from build123d import *

# Parameters (mm, degrees)
SKETCH_R   = 4.3
SKETCH_R_2 = 3.3
PAD_DEPTH  = 8


with BuildPart() as part:
    # Sketch → Pad (new body)
    with BuildSketch(Plane.XY):
        with BuildLine():
            Line((180, 10), (180, 490))
            ThreePointArc((180, 490), (177.071068, 497.071068), (170, 500))
            Line((10, 500), (170, 500))
            ThreePointArc((10, 500), (2.928932, 497.071068), (0, 490))
            Line((0, 490), (0, 10))
            ThreePointArc((0, 10), (2.928932, 2.928932), (10, 0))
            Line((10, 0), (170, 0))
            ThreePointArc((170, 0), (177.071068, 2.928932), (180, 10))
        make_face()
        with Locations((75, 318)):
            Circle(SKETCH_R, mode=Mode.SUBTRACT)
        with Locations((105, 318)):
            Circle(SKETCH_R, mode=Mode.SUBTRACT)
        with Locations((105, 299)):
            Circle(SKETCH_R, mode=Mode.SUBTRACT)
        with Locations((75, 299)):
            Circle(SKETCH_R, mode=Mode.SUBTRACT)
        with Locations((20, 20)):
            Circle(SKETCH_R_2, mode=Mode.SUBTRACT)
        with Locations((20, 75)):
            Circle(SKETCH_R_2, mode=Mode.SUBTRACT)
        with Locations((20, 130)):
            Circle(SKETCH_R_2, mode=Mode.SUBTRACT)
        with Locations((20, 185)):
            Circle(SKETCH_R_2, mode=Mode.SUBTRACT)
        with Locations((20, 480)):
            Circle(SKETCH_R_2, mode=Mode.SUBTRACT)
        with Locations((20, 425)):
            Circle(SKETCH_R_2, mode=Mode.SUBTRACT)
        with Locations((20, 370)):
            Circle(SKETCH_R_2, mode=Mode.SUBTRACT)
        with Locations((20, 315)):
            Circle(SKETCH_R_2, mode=Mode.SUBTRACT)
        with Locations((20, 240)):
            Circle(SKETCH_R_2, mode=Mode.SUBTRACT)
        with Locations((160, 480)):
            Circle(SKETCH_R_2, mode=Mode.SUBTRACT)
        with Locations((160, 425)):
            Circle(SKETCH_R_2, mode=Mode.SUBTRACT)
        with Locations((160, 370)):
            Circle(SKETCH_R_2, mode=Mode.SUBTRACT)
        with Locations((160, 315)):
            Circle(SKETCH_R_2, mode=Mode.SUBTRACT)
        with Locations((160, 240)):
            Circle(SKETCH_R_2, mode=Mode.SUBTRACT)
        with Locations((160, 20)):
            Circle(SKETCH_R_2, mode=Mode.SUBTRACT)
        with Locations((160, 75)):
            Circle(SKETCH_R_2, mode=Mode.SUBTRACT)
        with Locations((160, 130)):
            Circle(SKETCH_R_2, mode=Mode.SUBTRACT)
        with Locations((160, 185)):
            Circle(SKETCH_R_2, mode=Mode.SUBTRACT)
        with BuildLine():
            Line((65, 170), (115, 170))
            ThreePointArc((115, 170), (118.535534, 171.464466), (120, 175))
            Line((120, 287), (120, 175))
            ThreePointArc((120, 287), (118.535534, 290.535534), (115, 292))
            Line((65, 292), (115, 292))
            ThreePointArc((65, 292), (61.464466, 290.535534), (60, 287))
            Line((60, 175), (60, 287))
            ThreePointArc((60, 175), (61.464466, 171.464466), (65, 170))
        make_face(mode=Mode.SUBTRACT)
    extrude(amount=PAD_DEPTH)


solid = part.part
Check sheet for the modelled part. Datum: model origin and axes. Units: mm. A direction names the side the tool comes from. Give positions to 0.01 mm unless a question says otherwise; leave off trailing zeros. Write each loop counter-clockwise with the first axis right and the second up, starting at its lowest first coordinate (ties: lowest second). Pieces come first, ordered by that corner, then holes. Notation, with made-up numbers: (45, -13.5) -> (86, -13.5) arc R14 ccw to (86, -8.5) -> close; hole circle Ø9 at (62.25, 15.25). An arc over 180 degrees is marked (long way). One line per item, written item: value. Start each with the question number.
Item 1: Section check C-C on z = 1.75. State how many separate pieces and enclosed holes the cut face has, then the cut area to 3 significant figures.
Item 2: Gauge pin test, flat end, axial feed: pin 1 (7.5 mm diameter, centred on x = 20, y = 240, fed in from +Z). Record the tip position at first contact, or that the pin passes through.
Item 3: Draft check along Y on faces 3 (the flat face through (49, 254, 0)), 4 (the cylindrical face through (177.15, 496.99, 3.94)), 5 (the cylindrical face through (76.984, 314.185, 3.944)). Enter one of: +Y half, -Y half, draft (parallel to the pull), parting line (faces both ways), or undercut.
Item 4: Tool access check on faces 1 (the flat face through (49, 254, 8)), 2 (the flat face through (120, 232, 4)). Record the directions out of +Z, -Z, +X, -X, +Y, -Y that give a thin tool (end or side, any length) a straight path to the whole face; none if there is none.
Item 5: Material ranges on probe 1 along X at (y, z) = (425, 4); probe 2 along Y at (x, z) = (75, 4); probe 3 along X at (y, z) = (185, 4.25), recorded low to high. Write a range as from..to.
Item 6: Section check B-B on y = 299. Record the cut outline in (x, z), then the cut area to 3 significant figures.
Item 7: Section check A-A on x = 105. Record the cut outline in (y, z), then the cut area to 3 significant figures.
Results list:
1. separate pieces: 1
1. enclosed holes: 23
1. area: 81,800 mm²
2. pin 1: z = 8
3. face 3: draft
3. face 4: +Y half
3. face 5: undercut
4. face 1: +Z, +X, -X, +Y, -Y
4. face 2: +Z, -Z
5. probe 1: 0..16.7, 23.3..156.7, 163.3..180
5. probe 2: 0..170, 292..294.7, 303.3..313.7, 322.3..500
5. probe 3: 0..16.7, 23.3..60, 120..156.7, 163.3..180
6. outline: (0, 0) -> (70.7, 0) -> (70.7, 8) -> (0, 8) -> close; (79.3, 0) -> (100.7, 0) -> (100.7, 8) -> (79.3, 8) -> close; (109.3, 0) -> (180, 0) -> (180, 8) -> (109.3, 8) -> close
6. area: 1,300 mm²
7. outline: (0, 0) -> (170, 0) -> (170, 8) -> (0, 8) -> close; (292, 0) -> (294.7, 0) -> (294.7, 8) -> (292, 8) -> close; (303.3, 0) -> (313.7, 0) -> (313.7, 8) -> (303.3, 8) -> close; (322.3, 0) -> (500, 0) -> (500, 8) -> (322.3, 8) -> close
7. area: 2,890 mm²
